CAD build for the part. Positions are in the model's coordinates, mm. A direction names the side the tool comes from. Round coordinates to 2 decimals unless told otherwise and drop trailing zeros. Order: outer loops, then holes, each group sorted by start corner. A loop starts at its lowest first (then second) coordinate and runs counter-clockwise, first axis right, second up. Notation, with made-up numbers: M 30,49.5 L 87,49.5 A15 cw 87,61.5 Z; hole C 37.5,63 d2. An arc over 180 degrees is marked long. Answer as CSV lines item,"result". Start each with the question number.
```python
from build123d import *

# Parameters (mm, degrees)
SKETCH1_W           = 1828.8
SKETCH1_H           = 1219.2
BOSS_EXTRUDE1_DEPTH = 127
SKETCH2_W           = 1676.4
SKETCH2_H           = 1066.8
CUT_EXTRUDE2_DEPTH  = 101.6
SKETCH3_W           = 76.2
SKETCH3_H           = 50.8
BOSS_EXTRUDE2_DEPTH = 76.2
SKETCH4_W           = 76.2
SKETCH4_H           = 50.8
BOSS_EXTRUDE3_DEPTH = 76.2
SKETCH5_W           = 76.2
SKETCH5_H           = 50.8
BOSS_EXTRUDE4_DEPTH = 76.2


with BuildPart() as part:
    # Sketch1 → Boss-Extrude1 (new body)
    with BuildSketch(Plane.XY):
        with Locations((914.4, 609.6)):
            Rectangle(SKETCH1_W, SKETCH1_H)
    extrude(amount=BOSS_EXTRUDE1_DEPTH)

    # Sketch2 → Cut-Extrude2 (cut)
    with BuildSketch(Plane.XY.offset(127)):
        with Locations((914.4, 609.6)):
            Rectangle(SKETCH2_W, SKETCH2_H)
    extrude(amount=-CUT_EXTRUDE2_DEPTH, mode=Mode.SUBTRACT)

    # Sketch3 → Boss-Extrude2 (add)
    with BuildSketch(Plane.XY.offset(127)):
        with Locations((38.1, 1181.1)):
            Rectangle(SKETCH3_W, SKETCH3_H)
    extrude(amount=BOSS_EXTRUDE2_DEPTH)

    # Sketch4 → Boss-Extrude3 (add)
    with BuildSketch(Plane.XY.offset(127)):
        with Locations((1790.7, 1181.1)):
            Rectangle(SKETCH4_W, SKETCH4_H)
    extrude(amount=BOSS_EXTRUDE3_DEPTH)

    # Sketch5 → Boss-Extrude4 (add)
    with BuildSketch(Plane.XY.offset(127)):
        with Locations((38.1, 215.9)):
            Rectangle(SKETCH5_W, SKETCH5_H)
        with Locations((1790.7, 215.9)):
            Rectangle(SKETCH5_W, SKETCH5_H)
    extrude(amount=BOSS_EXTRUDE4_DEPTH)


solid = part.part
```
Q1. Drop flat-ended pins along their axis: P1, Ø23, axis at x = 1796, z = 153, coming from the -Y side; P2, Ø5, axis at x = 338, y = 1087.5, coming from the +Z side; P3, Ø23, axis at x = 1806, z = 169.5, coming from the +Y side. Give the stop position or say it passes through.
Q2. Band-saw the part on B-B, the plane x = 790. Write the cut outline in (y, z), then the cut area to 3 significant figures.
Q3. Probe line 1 along Y through (x, z) = (1364.5, 100.5); line 2 along X through (y, z) = (296.5, 44); line 3 along Z through (x, y) = (136.5, 88). List the from-to ranges inside material, lowest first. Write a range as from..to.
Q4. Mould opens along Y. For faces 5 (the flat face through (38, 1206.5, 165)), 6 (the flat face through (1790, 190.5, 165)), 7 (the flat face through (903, 1143, 77)) say: +Y half, -Y half, draft (parallel to the pull), parting line (faces both ways), or undercut.
Q5. Band-saw the part on C-C, the plane y = 1048.5. Write the cut outline in (x, z), then the cut area to 3 significant figures.
Q6. Tool access for faces 1 (the flat face through (1752.6, 1181, 165)), 2 (the flat face through (38, 190.5, 165)), 3 (the flat face through (903, 76.2, 77)), 4 (the flat face through (1790, 1206.5, 165)): list every direction of +Z, -Z, +X, -X, +Y, -Y with a clear straight run to the whole face (end or side of a thin tool).
Q7. Band-saw the part on A-A, the plane z = 148. Write the cut outline in (x, y).
Answer:
1,P1,"stops at y = 190.5"
1,P2,"stops at z = 25.4"
1,P3,"stops at y = 1206.5"
2,outline,"M 0,0 L 1219.2,0 L 1219.2,127 L 1143,127 L 1143,25.4 L 76.2,25.4 L 76.2,127 L 0,127 Z"
2,area,"46,500 mm^2"
3,line 1,"y = 0..76.2, 1143..1219.2"
3,line 2,"x = 0..76.2, 1752.6..1828.8"
3,line 3,"z = 0..25.4"
4,face 5,"+Y half"
4,face 6,"-Y half"
4,face 7,"undercut"
5,outline,"M 0,0 L 1828.8,0 L 1828.8,127 L 1752.6,127 L 1752.6,25.4 L 76.2,25.4 L 76.2,127 L 0,127 Z"
5,area,"61,900 mm^2"
6,face 1,"+Z, +Y, -Y"
6,face 2,"+Z, +X, -X, -Y"
6,face 3,"+Z"
6,face 4,"+Z, +X, -X, +Y"
7,outline,"M 0,190.5 L 76.2,190.5 L 76.2,241.3 L 0,241.3 Z; M 0,1155.7 L 76.2,1155.7 L 76.2,1206.5 L 0,1206.5 Z; M 1752.6,190.5 L 1828.8,190.5 L 1828.8,241.3 L 1752.6,241.3 Z; M 1752.6,1155.7 L 1828.8,1155.7 L 1828.8,1206.5 L 1752.6,1206.5 Z"
